Geometry: final body of the model. Coordinates: model frame, mm. Face numbers are marked on the shaded views. A direction names the side the tool comes from. Give positions to 0.01 mm unless a question says otherwise; leave off trailing zeros. Write each loop counter-clockwise with the first axis right and the second up, starting at its lowest first coordinate (ties: lowest second). Pieces come first, ordered by that corner, then holes. Notation, with made-up numbers: M -11,59.25 L 31,59.25 A32 cw 31,86.25 Z; hole C 79.25,0 d3. An arc over 180 degrees is marked long. Use a Markdown table: item, result. Add a question column.
1) Section B-B on y = 25. Return the cut outline in (x, z) (3 decimals).
2) Section A-A on z = -31. Return the cut outline in (x, y).
3) Section C-C on x = 11. Return the cut outline in (y, z) (3 decimals), then the cut area to 3 significant figures.
4) Pin query (flat end, axial travel): pin 1 (4 mm diameter, centred on x = 7, y = 35.5, fed in from -Z); pin 2 (10 mm diameter, centred on y = 20.5, z = -28, fed in from -X) (3 decimals); pin 3 (3 mm diameter, centred on y = 25, z = -3, fed in from +X); pin 4 (5 mm diameter, centred on x = 6.5, z = -20.5, fed in from +Y). Return the tip coordinate at first contact, or that it passes through.
5) Set-up query: the marked faces 5 and 6. Return all of +Z, -Z, +X, -X, +Y, -Y with unobstructed straight access to the full face (end or side cutting, diameter ignored); none if empty.
6) Section D-D on y = 32. Return the cut outline in (x, z).
7) Line query: line 1 (X direction, y = 7.5, z = -31); line 2 (X direction, y = 4.1, z = -31); line 3 (Y direction, x = 9.5, z = -4.5) (3 decimals). Output: solid intervals per line, ascending.
8) Draft query along X for the marked faces 1, 2, 3 and 4. Return one class per face: +X half, -X half, draft (parallel to the pull), parting line (faces both ways), or undercut.
```python
from build123d import *

# Parameters (mm, degrees)
PAD_DEPTH       = 15
SKETCH001_R     = 4.725
POCKET_DEPTH    = 28.285271
SKETCH002_W     = 13.497765
SKETCH002_H     = 2
POCKET001_DEPTH = 15.001
SKETCH007_W     = 9.919765
SKETCH007_H     = 5.5
SKETCH007_W_2   = 9.427402
POCKET002_DEPTH = 34
SKETCH008_W     = 17.002388
SKETCH008_H     = 12
POCKET003_DEPTH = 13
SKETCH009_R     = 4.75
POCKET004_DEPTH = 35.001
SKETCH010_W     = 8.09575
SKETCH010_H     = 1.5
POCKET005_DEPTH = 35.001
SKETCH011_R     = 1.4
POCKET006_DEPTH = 15.001
SKETCH012_R     = 1.4
POCKET007_DEPTH = 8
SKETCH013_R     = 1.75
POCKET008_DEPTH = 6.001
SKETCH014_R     = 1.875
POCKET009_DEPTH = 8


with BuildPart() as part:
    # Sketch → Pad (new body)
    with BuildSketch(Plane.YZ):
        Polygon((20.701614, 0), (40, 0), (40, -6), (34, -6), (5, -35), (0, -35), (0, -20.701614), align=None)
    extrude(amount=PAD_DEPTH)

    # Sketch001 (on Face4 of Pad) → Pocket (cut, through all)
    with BuildSketch(Plane(origin=(0, 20, -20), x_dir=(0, 0.707107, 0.707107), z_dir=(0, 0.707107, -0.707107))):
        with Locations((-32, 7.5)):
            Circle(SKETCH001_R)
    extrude(amount=-POCKET_DEPTH, mode=Mode.SUBTRACT)

    # Sketch002 (on Face8 of Pocket) → Pocket001 (cut, through all)
    with BuildSketch(Plane(origin=(0, 0, 0), x_dir=(0, 1, 0), z_dir=(-1, 0, 0))):
        with Locations((-21.822522, 7.5)):
            Rectangle(SKETCH002_W, SKETCH002_H)
    extrude(amount=-POCKET001_DEPTH, mode=Mode.SUBTRACT)

    # Sketch007 (on Face2 of Pocket001) → Pocket002 (cut)
    with BuildSketch(Plane.ZX.offset(40)):
        with Locations((-32.959882, 4)):
            Rectangle(SKETCH007_W, SKETCH007_H)
        with Locations((-32.713701, 11)):
            Rectangle(SKETCH007_W_2, SKETCH007_H)
    extrude(amount=-POCKET002_DEPTH, mode=Mode.SUBTRACT)

    # Sketch008 (on Face3 of Pocket002) → Pocket003 (cut)
    with BuildSketch(Plane.ZX.offset(40)):
        with Locations((-14.501194, 7.5)):
            Rectangle(SKETCH008_W, SKETCH008_H)
    extrude(amount=-POCKET003_DEPTH, mode=Mode.SUBTRACT)

    # Sketch009 (on Face1 of Pocket003) → Pocket004 (cut, through all)
    with BuildSketch(Plane(origin=(0, 0, 0), x_dir=(0, -1, 0), z_dir=(0, 0, 1))):
        with Locations((-32, 7.5)):
            Circle(SKETCH009_R)
    extrude(amount=-POCKET004_DEPTH, mode=Mode.SUBTRACT)

    # Sketch010 (on Face1 of Pocket004) → Pocket005 (cut, through all)
    with BuildSketch(Plane(origin=(0, 0, 0), x_dir=(0, -1, 0), z_dir=(0, 0, 1))):
        with Locations((-25.307632, 7.5)):
            Rectangle(SKETCH010_W, SKETCH010_H)
    extrude(amount=-POCKET005_DEPTH, mode=Mode.SUBTRACT)

    # Sketch011 (on Face3 of Pocket005) → Pocket006 (cut, through all)
    with BuildSketch(Plane(origin=(0, 0, 0), x_dir=(0, 1, 0), z_dir=(-1, 0, 0))):
        with Locations((25, 3)):
            Circle(SKETCH011_R)
    extrude(amount=-POCKET006_DEPTH, mode=Mode.SUBTRACT)

    # Sketch012 (on Face3 of Pocket006) → Pocket007 (cut)
    with BuildSketch(Plane(origin=(0, 0, 0), x_dir=(0, 1, 0), z_dir=(-1, 0, 0))):
        with Locations((25, 3)):
            Circle(SKETCH012_R)
    extrude(amount=-POCKET007_DEPTH, mode=Mode.SUBTRACT)

    # Sketch013 (on Face31 of Pocket007) → Pocket008 (cut, through all)
    with BuildSketch(Plane.ZX.offset(6)):
        with Locations((-31, 11)):
            Circle(SKETCH013_R)
        with Locations((-31, 4)):
            Circle(SKETCH013_R)
    extrude(amount=-POCKET008_DEPTH, mode=Mode.SUBTRACT)

    # Sketch014 (on Face4 of Pocket008) → Pocket009 (cut)
    with BuildSketch(Plane.YZ.offset(15)):
        with Locations((25, -3)):
            Circle(SKETCH014_R)
    extrude(amount=-POCKET009_DEPTH, mode=Mode.SUBTRACT)


solid = part.part
```
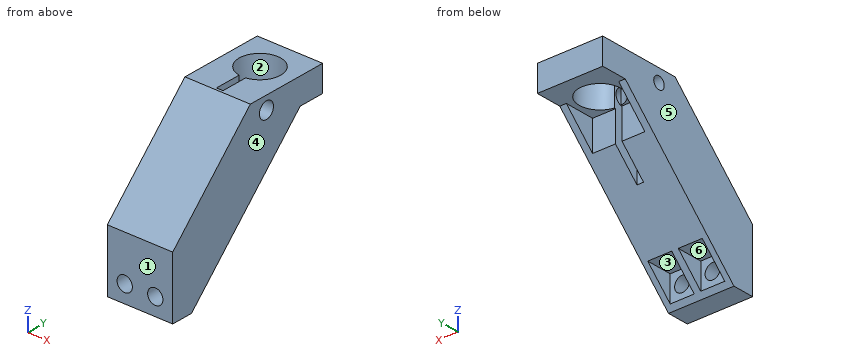
Found:
| question | item | result |
|---|---|---|
| 1 | outline | M 0,-15 L 6.75,-15 L 6.75,-4.4 L 0,-4.4 Z; M 0,-1.6 L 6.75,-1.6 L 6.75,0 L 0,0 Z; M 8.25,-15 L 15,-15 L 15,-4.875 L 8.25,-4.875 Z; M 8.25,-1.125 L 15,-1.125 L 15,0 L 8.25,0 Z |
| 2 | outline | M 0,0 L 2.25,0 L 2.25,6 L 1.25,6 L 1.25,9 L 0,9 Z; M 5.75,0 L 9.25,0 L 9.25,6 L 8.25,6 L 8.25,9 L 6.75,9 L 6.75,6 L 5.75,6 Z; M 12.75,0 L 15,0 L 15,9 L 13.75,9 L 13.75,6 L 12.75,6 Z |
| 3 | outline | M 0,-35 L 5,-35 L 6,-34 L 6,-32.75 L 0,-32.75 Z; M 0,-29.25 L 6,-29.25 L 6,-28 L 12,-28 L 27,-13 L 27,-6 L 28.789,-6 L 28.789,0 L 20.702,0 L 0,-20.702 Z; M 35.211,-6 L 40,-6 L 40,0 L 35.211,0 Z; hole C 25,-3 d3.75 |
| 3 | area | 478 mm² |
| 4 | pin 1 | z = -6 |
| 4 | pin 2 | through |
| 4 | pin 3 | x = 6.75 |
| 4 | pin 4 | y = 22 |
| 5 | face 5 | +Z, -Z, -X, +Y, -Y |
| 5 | face 6 | -Z, +Y |
| 6 | outline | M 0,-8 L 1.5,-8 L 1.5,-6 L 2.75,-6 L 2.75,0 L 0,0 Z; M 12.25,-6 L 13.5,-6 L 13.5,-8 L 15,-8 L 15,0 L 12.25,0 Z |
| 7 | line 1 | 0 to 1.25, 6.75 to 8.25, 13.75 to 15 |
| 7 | line 2 | 0 to 2.25, 5.75 to 9.25, 12.75 to 15 |
| 7 | line 3 | 16.202 to 23.875, 26.125 to 27.692, 36.308 to 40 |
| 8 | face 1 | draft |
| 8 | face 2 | undercut |
| 8 | face 3 | undercut |
| 8 | face 4 | +X half |
